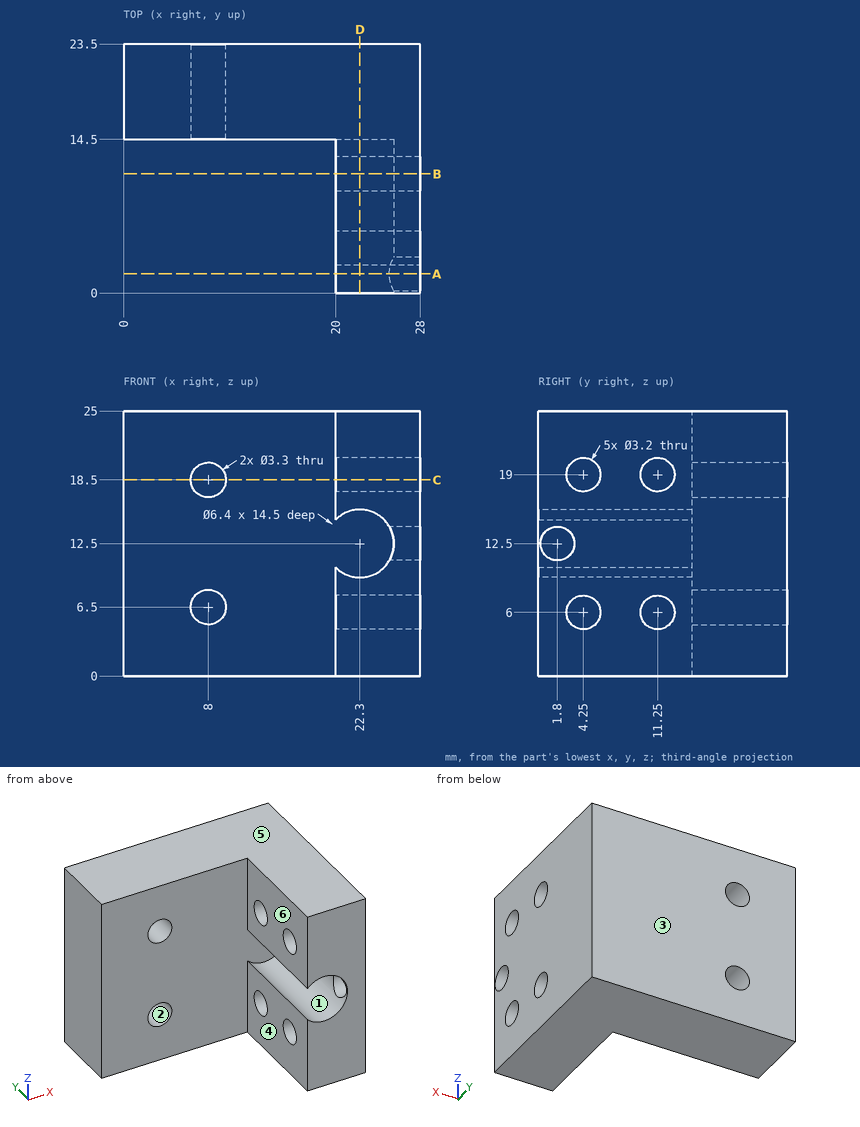
For this review, use the dimensioned drawing (mm, ordinates from the lowest corner) and the shaded views. A direction names the side the tool comes from. Give positions to 0.01 mm unless a question says otherwise; leave off trailing zeros. Order: outer loops, then holes, each group sorted by start corner. A loop starts at its lowest first (then second) coordinate and runs counter-clockwise, first axis right, second up. Notation, with made-up numbers: (39.5, 65) - (58.5, 65) arc R19 cw to (58.5, 97) - close; hole circle Ø5 at (69.25, 30). An arc over 180 degrees is marked (long way). Use a Markdown table: item, result. Add a question column.
(1) Add section A-A on y = 1.8. Give the boundary of the cut face in (x, z), then the cut area to 3 significant figures.
(2) Add section B-B on y = 11.25. Give the boundary of the cut face in (x, z).
(3) Machinability: for the marked faces 5 and 6, which of the approach directions +Z, -Z, +X, -X, +Y, -Y give a long, thin tool a straight path to every point of the face, cutting with its end or side? Answer none if there is none.
(4) Wall thickness on probe 1 along Z at (x, y) = (22.3, 4.25); probe 2 along Y at (x, z) = (13.75, 1.5); probe 3 along X at (y, z) = (11.25, 12.5): over which ranges is each line inside the solid? List them lowest first. Write a range as [from, to].
(5) Mouldability with a two-part tool opening along X and no side actions: class the marked faces 1, 2, 3 and 4 as +X half, -X half, draft (parallel to the pull), parting line (faces both ways), or undercut.
(6) Add section C-C on z = 18.5. Give the boundary of the cut face in (x, y).
(7) Clearance check with flat-ended pins moving along their axes: P1, Ø7.5, axis at x = 11, z = 17.5, coming from the -Y side; P2, Ø3, axis at y = 10.5, z = 20, coming from the -X side. State where each tip first meets the part, or that it passes through.
(8) Add section D-D on x = 22.3. Give the boundary of the cut face in (y, z), then the cut area to 3 significant figures.
Report:
| question | item | result |
|---|---|---|
| 1 | outline | (20, 0) - (28, 0) - (28, 10.9) - (25.07, 10.9) arc R3.2 cw to (20, 10.28) - close; (20, 14.72) arc R3.2 cw to (25.07, 14.1) - (28, 14.1) - (28, 25) - (20, 25) - close |
| 1 | area | 162 mm² |
| 2 | outline | (20, 0) - (28, 0) - (28, 4.4) - (20, 4.4) - close; (20, 7.6) - (28, 7.6) - (28, 17.4) - (20, 17.4) - (20, 14.72) arc R3.2 cw (long way) to (20, 10.28) - close; (20, 20.6) - (28, 20.6) - (28, 25) - (20, 25) - close |
| 3 | face 5 | +Z, +X, -X, +Y, -Y |
| 3 | face 6 | +Z, -Z, -X, -Y |
| 4 | probe 1 | z = [0, 4.4], [7.6, 9.3], [15.7, 17.4], [20.6, 25] |
| 4 | probe 2 | y = [14.5, 23.5] |
| 4 | probe 3 | x = [25.5, 28] |
| 5 | face 1 | undercut |
| 5 | face 2 | undercut |
| 5 | face 3 | draft |
| 5 | face 4 | -X half |
| 6 | outline | (0, 14.5) - (6.35, 14.5) - (6.35, 23.5) - (0, 23.5) - close; (9.65, 14.5) - (20, 14.5) - (20, 12.77) - (28, 12.77) - (28, 23.5) - (9.65, 23.5) - close; (20, 0) - (28, 0) - (28, 2.73) - (20, 2.73) - close; (20, 5.77) - (28, 5.77) - (28, 9.73) - (20, 9.73) - close |
| 7 | P1 | stops at y = 14.5 |
| 7 | P2 | stops at x = 20 |
| 8 | outline | (0, 0) - (23.5, 0) - (23.5, 25) - (0, 25) - (0, 15.7) - (14.5, 15.7) - (14.5, 9.3) - (0, 9.3) - close; hole circle Ø3.2 at (4.25, 6); hole circle Ø3.2 at (4.25, 19); hole circle Ø3.2 at (11.25, 6); hole circle Ø3.2 at (11.25, 19) |
| 8 | area | 463 mm² |
